```python
from build123d import *

# Parameters (mm, degrees)
F1_DEPTH      = 9
F2_R          = 4.5
F3_DEPTH      = 30
F4_W          = 85
F4_H          = 30
F5_DEPTH      = 25
F6_W          = 85
F6_H          = 30
F7_DEPTH      = 25
F9_R          = 1
F10_T1_DEPTH  = 277
F10_T3_DEPTH  = 190
F10_T5_DEPTH  = 48.1001500805
F10_T7_DEPTH  = 92.4223044172
F10_T10_ANGLE = 90
F10_T12_ANGLE = 90
F10_T14_ANGLE = 90
F10_T16_ANGLE = 90
F10_T18_ANGLE = 90
F10_T20_ANGLE = 90
F10_T22_ANGLE = 90
F10_T24_ANGLE = 90
F8_W          = 35
F8_H          = 75.194375382
F11_DEPTH     = 25


# Not quite as in the source:
# - a fillet or chamfer that OpenCascade refuses, or shapes differently, is made with other operations: its cross-section is extruded or revolved along the edge and cut away or added


with BuildPart() as f1:
    # F0 (on Front) → F1 (new body)
    with BuildSketch(Plane.XZ):
        with BuildLine():
            Line((131.9335396439, -4.1335214776), (-145.0664603561, -4.1335214776))
            ThreePointArc((-145.0664603561, -4.1335214776), (-152.137528168, -7.0624536657), (-155.0664603561, -14.1335214776))
            Line((-155.0664603561, -14.1335214776), (-155.0664603561, -204.1335214776))
            ThreePointArc((-155.0664603561, -204.1335214776), (-152.137528168, -211.2045892894), (-145.0664603561, -214.1335214776))
            Line((-145.0664603561, -214.1335214776), (131.9335396439, -214.1335214776))
            ThreePointArc((131.9335396439, -214.1335214776), (139.0046074557, -211.2045892894), (141.9335396439, -204.1335214776))
            Line((141.9335396439, -204.1335214776), (141.9335396439, -14.1335214776))
            ThreePointArc((141.9335396439, -14.1335214776), (139.0046074557, -7.0624536657), (131.9335396439, -4.1335214776))
        make_face()
    extrude(amount=F1_DEPTH)

    # F2 (on face) → F3 (join)
    with BuildSketch(Plane.XZ.offset(9)):
        with Locations((41.9335396439, -44.1335214776)):
            Circle(F2_R)
        with Locations((91.9335396439, -44.1335214776)):
            Circle(F2_R)
    extrude(amount=F3_DEPTH)

    # F4 (on face) → F5 (cut)
    with BuildSketch(Plane.XZ.offset(9)):
        with Locations((99.4335396439, -108.6974109549)):
            Rectangle(F4_W, F4_H)
    extrude(amount=-F5_DEPTH, mode=Mode.SUBTRACT)

    # F6 (on face) → F7 (cut)
    with BuildSketch(Plane.XZ.offset(9)):
        with Locations((99.4335396439, -153.8917863369)):
            Rectangle(F6_W, F6_H)
    extrude(amount=-F7_DEPTH, mode=Mode.SUBTRACT)

    # F9
    f9_edges = [f1.edges().sort_by_distance(p)[0] for p in [
        (37.43354, -39, -44.133521),
        (87.43354, -39, -44.133521),
    ]]
    fillet(f9_edges, radius=F9_R)

    # F10: chamfer of 5 on 2 edges, made by hand

    # F10_s2 → F10_t1 (cut)
    with BuildSketch(Plane.YZ.offset(-145.0664603561)):
        Polygon((-9, -9.1335214776), (-4, -4.1335214776), (-9, -4.1335214776), align=None)
        Polygon((-5, -4.1335214776), (0, -9.1335214776), (0, -4.1335214776), align=None)
        Polygon((-5, -214.1335214776), (0, -209.1335214776), (0, -214.1335214776), align=None)
        Polygon((-9, -209.1335214776), (-4, -214.1335214776), (-9, -214.1335214776), align=None)
    extrude(amount=F10_T1_DEPTH, mode=Mode.SUBTRACT)

    # F10_s4 → F10_t3 (cut)
    with BuildSketch(Plane.XY.offset(-204.1335214776)):
        Polygon((-155.0664603561, -5), (-150.0664603561, 0), (-155.0664603561, 0), align=None)
        Polygon((-150.0664603561, -9), (-155.0664603561, -4), (-155.0664603561, -9), align=None)
    extrude(amount=F10_T3_DEPTH, mode=Mode.SUBTRACT)

    # F10_s6 → F10_t5 (cut)
    with BuildSketch(Plane.XY.offset(-204.1335214776)):
        Polygon((141.9335396439, -5), (136.9335396439, 0), (141.9335396439, 0), align=None)
        Polygon((136.9335396439, -9), (141.9335396439, -4), (141.9335396439, -9), align=None)
    extrude(amount=F10_T5_DEPTH, mode=Mode.SUBTRACT)

    # F10_s8 → F10_t7 (cut)
    with BuildSketch(Plane.XY.offset(-106.5558258947)):
        Polygon((141.9335396439, -5), (136.9335396439, 0), (141.9335396439, 0), align=None)
        Polygon((136.9335396439, -9), (141.9335396439, -4), (141.9335396439, -9), align=None)
    extrude(amount=F10_T7_DEPTH, mode=Mode.SUBTRACT)

    # F10_s9 → F10_t10 (revolve, cut)
    with BuildSketch(Plane.XY.offset(-14.1335214776)):
        Polygon((141.9335396439, -5), (136.9335396439, 0), (141.9335396439, 0), align=None)
    revolve(axis=Axis((131.9335396439, 0, -14.1335214776), (0, -1, 0)), revolution_arc=F10_T10_ANGLE, mode=Mode.SUBTRACT)

    # F10_s11 → F10_t12 (revolve, cut)
    with BuildSketch(Plane.YZ.offset(-145.0664603561)):
        Polygon((-5, -4.1335214776), (0, -9.1335214776), (0, -4.1335214776), align=None)
    revolve(axis=Axis((-145.0664603561, 0, -14.1335214776), (0, -1, 0)), revolution_arc=F10_T12_ANGLE, mode=Mode.SUBTRACT)

    # F10_s13 → F10_t14 (revolve, cut)
    with BuildSketch(Plane.XY.offset(-204.1335214776)):
        Polygon((-155.0664603561, -5), (-150.0664603561, 0), (-155.0664603561, 0), align=None)
    revolve(axis=Axis((-145.0664603561, 0, -204.1335214776), (0, -1, 0)), revolution_arc=F10_T14_ANGLE, mode=Mode.SUBTRACT)

    # F10_s15 → F10_t16 (revolve, cut)
    with BuildSketch(Plane.YZ.offset(131.9335396439)):
        Polygon((-5, -214.1335214776), (0, -209.1335214776), (0, -214.1335214776), align=None)
    revolve(axis=Axis((131.9335396439, 0, -204.1335214776), (0, -1, 0)), revolution_arc=F10_T16_ANGLE, mode=Mode.SUBTRACT)

    # F10_s17 → F10_t18 (revolve, cut)
    with BuildSketch(Plane.XY.offset(-14.1335214776)):
        Polygon((136.9335396439, -9), (141.9335396439, -4), (141.9335396439, -9), align=None)
    revolve(axis=Axis((131.9335396439, -9, -14.1335214776), (0, -1, 0)), revolution_arc=F10_T18_ANGLE, mode=Mode.SUBTRACT)

    # F10_s19 → F10_t20 (revolve, cut)
    with BuildSketch(Plane.YZ.offset(-145.0664603561)):
        Polygon((-9, -9.1335214776), (-4, -4.1335214776), (-9, -4.1335214776), align=None)
    revolve(axis=Axis((-145.0664603561, -9, -14.1335214776), (0, -1, 0)), revolution_arc=F10_T20_ANGLE, mode=Mode.SUBTRACT)

    # F10_s21 → F10_t22 (revolve, cut)
    with BuildSketch(Plane.XY.offset(-204.1335214776)):
        Polygon((-150.0664603561, -9), (-155.0664603561, -4), (-155.0664603561, -9), align=None)
    revolve(axis=Axis((-145.0664603561, -9, -204.1335214776), (0, -1, 0)), revolution_arc=F10_T22_ANGLE, mode=Mode.SUBTRACT)

    # F10_s23 → F10_t24 (revolve, cut)
    with BuildSketch(Plane.YZ.offset(131.9335396439)):
        Polygon((-9, -209.1335214776), (-4, -214.1335214776), (-9, -214.1335214776), align=None)
    revolve(axis=Axis((131.9335396439, -9, -204.1335214776), (0, -1, 0)), revolution_arc=F10_T24_ANGLE, mode=Mode.SUBTRACT)

    # F8 (on face) → F11 (cut)
    with BuildSketch(Plane.XZ.offset(9)):
        with Locations((29.6793225408, -131.2945986459)):
            Rectangle(F8_W, F8_H)
    extrude(amount=-F11_DEPTH, mode=Mode.SUBTRACT)


solid = f1.part
```
Read the model definition and answer for the solid it produces. Units are mm, in the model's axes. A direction names the side the tool comes from. Coordinates: 2 decimals unless noted, no trailing zeros. Write each loop counter-clockwise with the first axis right and the second up, starting at its lowest first coordinate (ties: lowest second). Pieces come first, ordered by that corner, then holes. Notation, with made-up numbers: (4, 76.25) - (53, 76.25) arc R19 cw to (53, 111.25) - close; hole circle Ø3 at (-10, -27). An arc over 180 degrees is marked (long way). Answer as a JSON object with one key per item and string values. Group by question number.
1. A cutting plane is placed at B-B (x = -103.5). Determine the outline of the cut face in (y, z).
2. A cutting plane is placed at A-A (z = -116). Determine the outline of the cut face in (x, y).
3. Which of the six approach directions +Z, -Z, +X, -X, +Y, -Y give full straight-line access (tool end or side, diameter ignored) to faces 1 (the flat face through (99, -5, -168.892)), 2 (the flat face through (29, -5, -93.697)), 3 (the cylindrical face through (40.958, -23.297, -48.527))?
4. The mould has two halves that part along X. Classify faces 4 (the flat face through (99, -5, -93.697)), 5 (the cylindrical face through (90.958, -23.297, -48.527)), 6 (the conical face through (-149.91, -7.22, -208.88)): +X half, -X half, draft (parallel to the pull), parting line (faces both ways), or undercut.
5. A cutting plane is placed at C-C (z = -193). Determine the outline of the cut face in (x, y).
6. Consider L1, parallel to Y at x = -119, z = -177; L2, parallel to Z at x = 130, y = -2; L3, parallel to X at y = -7, z = -22. Determine where each line is inside the solid, lowest interval first. Write a range as [from, to].
7. Each of these flat-tipped pins is pushed along its axis until it touches: P1, Ø6, axis at y = -8.5, z = -27.5, coming from the -X side; P2, Ø7, axis at y = -5, z = -146, coming from the +X side; P3, Ø6, axis at x = -86.5, y = -8.5, coming from the +Z side. Where does it stop, or does it pass through?
8. A cutting plane is placed at D-D (y = -15). Determine the outline of the cut face in (x, z).
Worked out:
{
 "1": {"outline": "(-9, -209.13) - (-4.5, -213.63) - (0, -209.13) - (0, -9.13) - (-4.5, -4.63) - (-9, -9.13) - close"},
 "2": {"outline": "(-154.57, -4.5) - (-150.07, -9) - (12.18, -9) - (12.18, 0) - (-150.07, 0) - close; (47.18, -9) - (56.93, -9) - (56.93, 0) - (47.18, 0) - close"},
 "3": {"face 1": "+X, +Y, -Y", "face 2": "+Y, -Y", "face 3": "-Y"},
 "4": {"face 4": "draft", "face 5": "undercut", "face 6": "-X half"},
 "5": {"outline": "(-154.57, -4.5) - (-150.07, -9) - (136.93, -9) - (141.43, -4.5) - (136.93, 0) - (-150.07, 0) - close"},
 "6": {"L1": "y = [-9, 0]", "L2": "z = [-211.13, -168.89], [-138.89, -123.7], [-93.7, -7.13]", "L3": "x = [-152.07, 138.93]"},
 "7": {"P1": "stops at x = -153.57", "P2": "stops at x = 56.93", "P3": "stops at z = -5.63"},
 "8": {"outline": "circle Ø9 at (41.93, -44.13); circle Ø9 at (91.93, -44.13)"}
}
